from build123d import *

# Parameters (mm, degrees)
F1_DEPTH = 15
F2_R     = 2.5
F3_DEPTH = 10
F4_R     = 2


with BuildPart() as f1:
    # F0 (on Top) → F1 (new body)
    with BuildSketch(Plane.XY):
        with BuildLine():
            Line((34, 16), (-34, 16))
            ThreePointArc((-34, 16), (-34.707107, 15.707107), (-35, 15))
            Line((-35, 15), (-35, -15))
            ThreePointArc((-35, -15), (-34.707107, -15.707107), (-34, -16))
            Line((-34, -16), (34, -16))
            ThreePointArc((34, -16), (34.707107, -15.707107), (35, -15))
            Line((35, -15), (35, 15))
            ThreePointArc((35, 15), (34.707107, 15.707107), (34, 16))
        make_face()
    extrude(amount=-F1_DEPTH)

    # F2 (on face) → F3 (join)
    with BuildSketch(Plane.XY):
        with Locations((-19.5, 0)):
            Circle(F2_R)
        with Locations((-6.5, 0)):
            Circle(F2_R)
        with Locations((6.5, 0)):
            Circle(F2_R)
        with Locations((19.5, 0)):
            Circle(F2_R)
    extrude(amount=F3_DEPTH)

    # F4
    f4_edges = [f1.edges().sort_by_distance(p)[0] for p in [
        (17, 0, 10),
        (4, 0, 10),
        (-9, 0, 10),
        (-22, 0, 10),
    ]]
    fillet(f4_edges, radius=F4_R)


solid = f1.part
Work out the finished part from the listing and answer in its coordinate system (mm). A direction names the side the tool comes from. Round coordinates to 2 decimals unless told otherwise and drop trailing zeros. Loops run counter-clockwise (first coordinate to the right, second up) from the corner with the lowest first, then second, coordinate; pieces in that order, holes last. Notation, with made-up numbers: (-33, -27) -> (-22, -27) arc R25 cw to (-22, 6) -> close; hole circle Ø5 at (-27.75, 44.5). An arc over 180 degrees is marked (long way). Use one line per item in the form item = value.
(1) For a pull along X with two mould halves and no side action, classify faces 1 (the flat face through (-35, 0, -7)), 2 (the cylindrical face through (-4.115, 0.751, 3.944)), 3 (the flat face through (0, -16, -7)) as released by +X, released by -X, zero draft, split by the parting line, or undercut.
Answer list:
face_1 = released by -X
face_2 = undercut
face_3 = zero draft
(2) A tool of negligible diameter and unlimited length cuts with its end or side. For faces 4 (the flat face through (0, 16, -7)), 5 (the cylindrical face through (-22, 0, 4)), from which of +Z, -Z, +X, -X, +Y, -Y can it reach the whole face along a straight path? Write none if from no direction.
Answer list:
face_4 = +Z, -Z, +X, -X, +Y
face_5 = +Z
(3) Find section C-C on y = -11. Give the vertices of the cut face in (x, z).
Answer list:
outline = (-35, -15) -> (35, -15) -> (35, 0) -> (-35, 0) -> close
(4) Find section B-B on x = -25. Give the vertices of the cut face in (y, z), then the cut area to 3 significant figures.
Answer list:
outline = (-16, -15) -> (16, -15) -> (16, 0) -> (-16, 0) -> close
area = 480 mm2
(5) Find section A-A on z = 6.5. Give the vertices of the cut face in (x, y), then the cut area to 3 significant figures.
Answer list:
outline = circle Ø5 at (-19.5, 0); circle Ø5 at (-6.5, 0); circle Ø5 at (6.5, 0); circle Ø5 at (19.5, 0)
area = 78.5 mm2
(6) Straight lines are drawn through the part: line 1 (X direction, y = 1.5, z = 1); line 2 (Z direction, x = -4, y = 6); line 3 (X direction, y = -0.5, z = 5.25). For each, find the intervals that lie inside material, in ascending order.
Answer list:
line_1 = -21.5 to -17.5, -8.5 to -4.5, 4.5 to 8.5, 17.5 to 21.5
line_2 = -15 to 0
line_3 = -21.95 to -17.05, -8.95 to -4.05, 4.05 to 8.95, 17.05 to 21.95
(7) Flat-ended cylindrical pins translate along their axes: P1, Ø3, axis at y = -2.5, z = 3, coming from the +X side; P2, Ø4, axis at x = 2, y = 3.5, coming from the +Z side. Find the tip coordinate at first contact, or state that the pin passes through.
Answer list:
P1 = 21.79
P2 = 0
